Can you work these out from the model? Positions are in its coordinate system, mm. A direction names the side the tool comes from. Give positions to 0.01 mm unless a question says otherwise; leave off trailing zeros. Loops run counter-clockwise (first coordinate to the right, second up) from the corner with the lowest first, then second, coordinate; pieces in that order, holes last. Notation, with made-up numbers: (0.25, -30) - (54.25, -30) arc R9 ccw to (54.25, -13) - close; hole circle Ø7 at (-17.5, -25.5). An arc over 180 degrees is marked (long way). Answer as a JSON object with one key per item and string values.
```python
from build123d import *

# Parameters (mm, degrees)
F0_R     = 1.7272
F0_R_2   = 9.525
F0_R_3   = 26.67
F1_DEPTH = 3.175
F2_R     = 4.7625


with BuildPart() as f1:
    # F0 (on Top) → F1 (new body)
    with BuildSketch(Plane.XY):
        with BuildLine():
            Line((66.6623, 36.195), (-66.6623, 36.195))
            Line((-66.6623, 36.195), (-66.6623, -35.3695))
            Line((-66.6623, -35.3695), (-47.6123, -35.3695))
            Line((-47.6123, -35.3695), (-13.812487, -65.816176))
            ThreePointArc((-13.812487, -65.816176), (0, -71.12), (13.812487, -65.816176))
            Line((13.812487, -65.816176), (47.6123, -35.3695))
            Line((47.6123, -35.3695), (66.6623, -35.3695))
            Line((66.6623, -35.3695), (66.6623, 36.195))
        make_face()
        with Locations((-11.786586, -62.269086)):
            Circle(F0_R, mode=Mode.SUBTRACT)
        with Locations((-61.8998, -30.607)):
            Circle(F0_R, mode=Mode.SUBTRACT)
        with Locations((-52.3748, -30.607)):
            Circle(F0_R, mode=Mode.SUBTRACT)
        with Locations((-11.786586, -38.695914)):
            Circle(F0_R, mode=Mode.SUBTRACT)
        with Locations((-22.226134, -22.226134)):
            Circle(F0_R, mode=Mode.SUBTRACT)
        with Locations((11.786586, -62.269086)):
            Circle(F0_R, mode=Mode.SUBTRACT)
        with Locations((0, -50.4825)):
            Circle(F0_R_2, mode=Mode.SUBTRACT)
        with Locations((11.786586, -38.695914)):
            Circle(F0_R, mode=Mode.SUBTRACT)
        with Locations((22.226134, -22.226134)):
            Circle(F0_R, mode=Mode.SUBTRACT)
        with Locations((52.3748, -30.607)):
            Circle(F0_R, mode=Mode.SUBTRACT)
        with Locations((61.8998, -30.607)):
            Circle(F0_R, mode=Mode.SUBTRACT)
        with Locations((-61.8998, 31.4325)):
            Circle(F0_R, mode=Mode.SUBTRACT)
        with Locations((-52.3748, 30.607)):
            Circle(F0_R, mode=Mode.SUBTRACT)
        with Locations((-22.226134, 22.226134)):
            Circle(F0_R, mode=Mode.SUBTRACT)
        Circle(F0_R_3, mode=Mode.SUBTRACT)
        with Locations((22.226134, 22.226134)):
            Circle(F0_R, mode=Mode.SUBTRACT)
        with Locations((52.3748, 30.607)):
            Circle(F0_R, mode=Mode.SUBTRACT)
        with Locations((61.8998, 31.4325)):
            Circle(F0_R, mode=Mode.SUBTRACT)
    extrude(amount=F1_DEPTH)

    # F2
    f2_edges = [f1.edges().sort_by_distance(p)[0] for p in [
        (-66.6623, 36.195, 1.5875),
        (66.6623, 36.195, 1.5875),
        (66.6623, -35.3695, 1.5875),
        (-66.6623, -35.3695, 1.5875),
    ]]
    fillet(f2_edges, radius=F2_R)


solid = f1.part
```
1) If we mould it in two halves opening along Y, with no side actions, what happens to faces 1 (the flat face through (-30.95, -50.38, 1.57)), 2 (the cylindrical face through (-63.625, 31.508, 1.565)), 3 (the cylindrical face through (65.23, 34.837, 1.61))? For each: released by +Y, released by -Y, zero draft, split by the parting line, or undercut.
Check sheet entries:
{"face 1": "released by -Y", "face 2": "undercut", "face 3": "released by +Y"}
2) I need wall thicknesses on L1, parallel to X at y = -22, z = 1.6; L2, parallel to Y at x = -12, z = 0.75 (3 decimals); L3, parallel to Y at x = -8, z = 2.95 (3 decimals). Which ranges of each line are inside material? Lowest first, please.
Check sheet entries:
{"L1": "-66.66 to -23.94, -20.51 to -15.08, 15.08 to 20.51, 23.94 to 66.66", "L2": "-67.273 to -63.983, -60.555 to -40.41, -36.982 to -23.818, 23.818 to 36.195", "L3": "-69.506 to -55.652, -45.313 to -25.442, 25.442 to 36.195"}
3) Imagine slicing it at A-A on x = 0. Write out the boundary of the cut face in (y, z) (1 decimal).
Check sheet entries:
{"outline": "(-71.1, 0) - (-60, 0) - (-60, 3.2) - (-71.1, 3.2) - close; (-41, 0) - (-26.7, 0) - (-26.7, 3.2) - (-41, 3.2) - close; (26.7, 0) - (36.2, 0) - (36.2, 3.2) - (26.7, 3.2) - close"}
4) Imagine slicing it at B-B on y = 0. Write out the boundary of the cut face in (x, z) (3 decimals), and give its area (3 significant figures).
Check sheet entries:
{"outline": "(-66.662, 0) - (-26.67, 0) - (-26.67, 3.175) - (-66.662, 3.175) - close; (26.67, 0) - (66.662, 0) - (66.662, 3.175) - (26.67, 3.175) - close", "area": "254 mm2"}
5) Imagine slicing it at D-D on z = 1.95. Give the number of separate pieces and of enclosed holes in the cut face, and give its area (3 significant figures).
Check sheet entries:
{"separate pieces": "1", "enclosed holes": "18", "area": "8,820 mm2"}
6) Which directions (+Z, -Z, +X, -X, +Y, -Y) give clear straight access to the entire face, cutting with the end or side of a thin tool? Please do faces 4 (the cylindrical face through (-65.23, 34.837, 1.61)), 5 (the flat face through (-55, -35.37, 2)).
Check sheet entries:
{"face 4": "+Z, -Z, -X, +Y", "face 5": "+Z, -Z, -X, -Y"}
7) I'm going to push flat-ended pins straight in: P1, Ø1, axis at x = 48.5, z = 1.5, coming from the -Y side; P2, Ø1.5, axis at x = 6.5, z = 0.5, coming from the -Y side. Where does each tip first touch, or does it pass through?
Check sheet entries:
{"P1": "y = -35.37", "P2": "y = -70.3"}
8) Imagine slicing it at C-C on x = -19. Write out the boundary of the cut face in (y, z) (3 decimals).
Check sheet entries:
{"outline": "(-61.143, 0) - (-18.716, 0) - (-18.716, 3.175) - (-61.143, 3.175) - close; (18.716, 0) - (36.195, 0) - (36.195, 3.175) - (18.716, 3.175) - close"}
